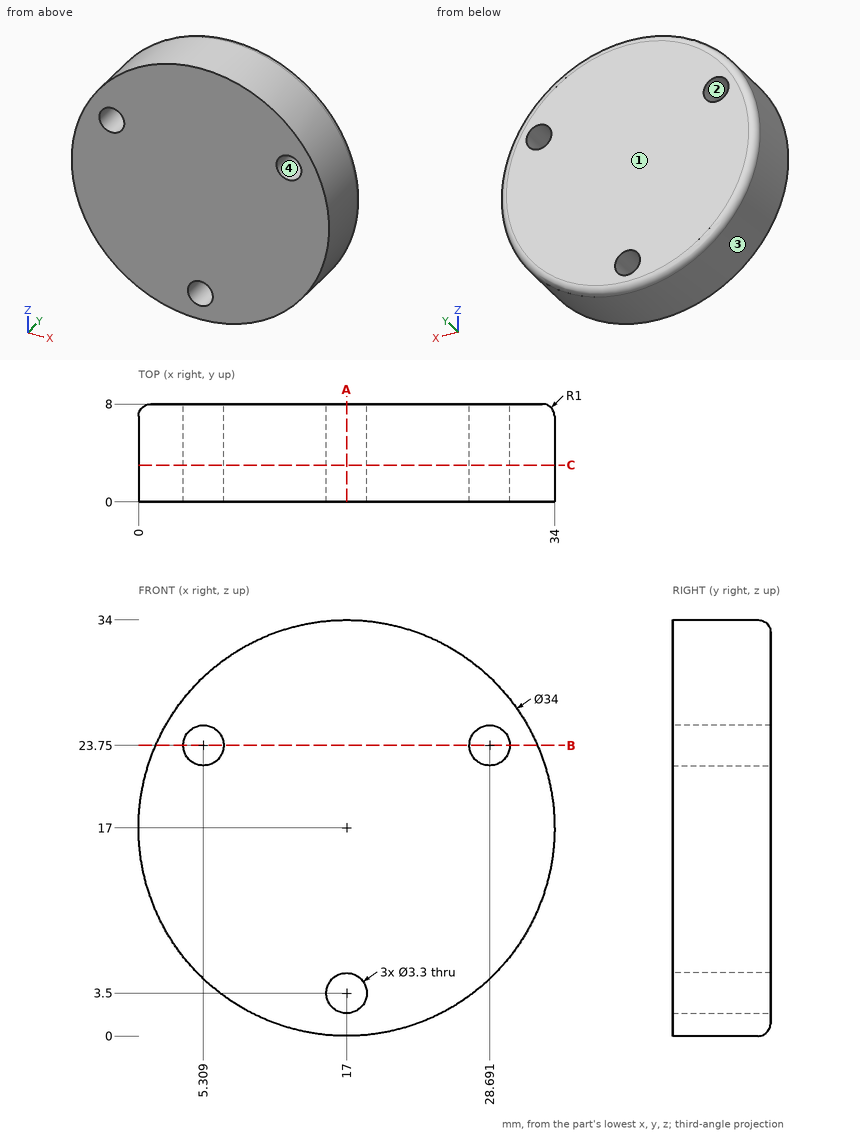
Geometry: see drawing. Coordinates: mm, zero at the bounding-box minimum. Coordinates: 2 decimals unless noted, no trailing zeros. Order: outer loops, then holes, each group sorted by start corner. A loop starts at its lowest first (then second) coordinate and runs counter-clockwise, first axis right, second up. Notation, with made-up numbers: (49, -4.5) - (99, -4.5) arc R31 ccw to (99, 33.5) - close; hole circle Ø10 at (-5, 3). An arc over 180 degrees is marked (long way). Return JSON: item names as keys, results as strings.
Q1. Cut plane C-C (y = 3). Return loops of the section in (x, z).
The answers:
{"outline": "circle Ø34 at (17, 17); hole circle Ø3.3 at (5.31, 23.75); hole circle Ø3.3 at (17, 3.5); hole circle Ø3.3 at (28.69, 23.75)"}
Q2. Cut plane A-A (x = 17). Return loops of the section in (y, z), then the cut area to 3 significant figures.
The answers:
{"outline": "(0, 0) - (7, 0) arc R1 ccw to (8, 1) - (8, 1.85) - (0, 1.85) - close; (0, 5.15) - (8, 5.15) - (8, 33) arc R1 ccw to (7, 34) - (0, 34) - close", "area": "245 mm2"}
Q3. First-contact query: pin 1 (1.5 mm diameter, centred on y = 3, z = 10, fed in from -X); pin 2 (1.5 mm diameter, centred on x = 16, y = 1.5, fed in from -Z); pin 3 (2 mm diameter, centred on y = 3.5, z = 23, fed in from -X). Flat tips, straight axial feed; report the tip coordinate or a pass-through.
The answers:
{"pin 1": "stops at x = 1.19", "pin 2": "stops at z = 0", "pin 3": "stops at x = 0.75"}
Q4. Draft query along Z for the marked faces 1, 2, 3 and 4. Return one class per face: +Z half, -Z half, draft (parallel to the pull), parting line (faces both ways), or undercut.
The answers:
{"face 1": "draft", "face 2": "undercut", "face 3": "parting line", "face 4": "undercut"}
Q5. Ray query, probe 1 along X at (y, z) = (2.5, 23.75); probe 2 along Z at (x, y) = (18.5, 3.5) (1 decimal); probe 3 along Z at (x, y) = (29.5, 1.5). Return the intervals inside material, ascending.
The answers:
{"probe 1": "x = 1.4 to 3.66, 6.96 to 27.04, 30.34 to 32.6", "probe 2": "z = 0.1 to 2.8, 4.2 to 33.9", "probe 3": "z = 5.48 to 22.31, 25.19 to 28.52"}
Q6. Cut plane B-B (z = 23.75). State how many separate pieces and enclosed holes the cut face has, then the cut area to 3 significant figures.
The answers:
{"separate pieces": "3", "enclosed holes": "0", "area": "196 mm2"}
